The listing builds one solid part. Answer for the finished solid, in the listing's coordinates (mm). Face numbers are marked on the shaded views. A direction names the side the tool comes from. Coordinates: 2 decimals unless noted, no trailing zeros. Order: outer loops, then holes, each group sorted by start corner. A loop starts at its lowest first (then second) coordinate and runs counter-clockwise, first axis right, second up. Notation, with made-up numbers: (66, 89.25) -> (92, 89.25) arc R21 ccw to (92, 125.25) -> close; hole circle Ø5 at (-31, -26). An arc over 180 degrees is marked (long way). Answer in a Markdown table with one row per item. Add a question column.
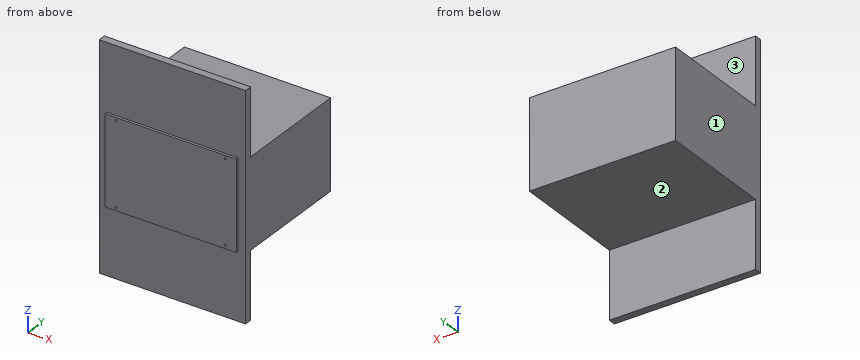
```python
from build123d import *

# Parameters (mm, degrees)
ESQUISSE1_W             = 590
ESQUISSE1_H             = 500
BOSS_EXTRU_1_DEPTH      = 360
ESQUISSE2_W             = 530
ESQUISSE2_H             = 360
BOSS_EXTRU_2_DEPTH      = 10
ESQUISSE3_R             = 4
ENL_V_MAT_EXTRU_1_DEPTH = 10
ESQUISSE4_W             = 590
ESQUISSE4_H             = 30
BOSS_EXTRU_3_DEPTH      = 270
BOSS_EXTRU_4_START      = -360
ESQUISSE4_2_W           = 590
ESQUISSE4_2_H           = 30
BOSS_EXTRU_4_DEPTH      = 270


with BuildPart() as part:
    # Esquisse1 → Boss.-Extru.1 (new body)
    with BuildSketch(Plane.XY):
        with Locations((295, 250)):
            Rectangle(ESQUISSE1_W, ESQUISSE1_H)
    extrude(amount=BOSS_EXTRU_1_DEPTH)

    # Esquisse2 → Boss.-Extru.2 (add)
    with BuildSketch(Plane.XZ):
        with Locations((295, 180)):
            Rectangle(ESQUISSE2_W, ESQUISSE2_H)
    extrude(amount=BOSS_EXTRU_2_DEPTH)

    # Esquisse3 → Enlèv. mat.-Extru.1 (cut)
    with BuildSketch(Plane.XZ.offset(10)):
        with Locations(Location((75, 12.5, 0), (0, 0, 270))):
            Circle(ESQUISSE3_R)
        with Locations(Location((515, 12.5, 0), (0, 0, 270))):
            Circle(ESQUISSE3_R)
        with Locations(Location((515, 347.5, 0), (0, 0, 270))):
            Circle(ESQUISSE3_R)
        with Locations(Location((75, 347.5, 0), (0, 0, 270))):
            Circle(ESQUISSE3_R)
    extrude(amount=-ENL_V_MAT_EXTRU_1_DEPTH, mode=Mode.SUBTRACT)

    # Esquisse4 → Boss.-Extru.3 (add)
    with BuildSketch(Plane.XY.offset(360)):
        with Locations((295, 15)):
            Rectangle(ESQUISSE4_W, ESQUISSE4_H)
    extrude(amount=BOSS_EXTRU_3_DEPTH)

    # Esquisse4<2> → Boss.-Extru.4 (add)
    with BuildSketch(Plane.XY.offset(360).offset(BOSS_EXTRU_4_START)):
        with Locations((295, 15)):
            Rectangle(ESQUISSE4_2_W, ESQUISSE4_2_H)
    extrude(amount=-BOSS_EXTRU_4_DEPTH)


solid = part.part
```
Q1. A cutting plane is placed at A-A (x = 133). Determine the outline of the cut face in (y, z).
Q2. Straight lines are drawn through the part: line 1 (Z direction, x = 515, y = -4); line 2 (X direction, y = -7.75, z = 12.5); line 3 (Z direction, x = 508, y = 292). For each, find the intervals that lie inside material, in ascending order.
Q3. A cutting plane is placed at B-B (y = 429). Determine the outline of the cut face in (x, z), then the cut area to 3 significant figures.
Q4. Given pin 1 (2.5 mm diameter, centred on x = 76.5, z = 11, fed in from -Y); pin 2 (5 mm diameter, centred on x = 337.5, y = 274, fed in from -Z); pin 3 (1.5 mm diameter, centred on x = 135, y = 290.5, fed in from +Z), each flat-ended and moving along its own axis, determine where each tip first touches the part or whether it passes through.
Q5. A cutting plane is placed at C-C (z = 501). Determine the outline of the cut face in (x, y).
Q6. For the marked faces 1, 2 and 3, determine the directions among +Z, -Z, +X, -X, +Y, -Y from which every point of the face is accessible in a straight line to the end or side of a thin tool.
Returned:
| question | item | result |
|---|---|---|
| 1 | outline | (-10, 0) -> (0, 0) -> (0, -270) -> (30, -270) -> (30, 0) -> (500, 0) -> (500, 360) -> (30, 360) -> (30, 630) -> (0, 630) -> (0, 360) -> (-10, 360) -> close |
| 2 | line 1 | z = 0 to 8.5, 16.5 to 343.5, 351.5 to 360 |
| 2 | line 2 | x = 30 to 71, 79 to 511, 519 to 560 |
| 2 | line 3 | z = 0 to 360 |
| 3 | outline | (0, 0) -> (590, 0) -> (590, 360) -> (0, 360) -> close |
| 3 | area | 212,000 mm² |
| 4 | pin 1 | stops at y = 0 |
| 4 | pin 2 | stops at z = 0 |
| 4 | pin 3 | stops at z = 360 |
| 5 | outline | (0, 0) -> (590, 0) -> (590, 30) -> (0, 30) -> close |
| 6 | face 1 | +Z, -Z, -X, +Y, -Y |
| 6 | face 2 | -Z, +X, -X, +Y |
| 6 | face 3 | +Z, +X, -X, +Y |
